Autodesk Inventor part; units mm, degrees
ref_plane "YZ Plane" through (0, 0, 0) normal (1, 0, 0) x (0, 1, 0)
ref_plane "XZ Plane" through (0, 0, 0) normal (0, 1, 0) x (-1, 0, 0)
ref_plane "XY Plane" through (0, 0, 0) normal (0, 0, 1) x (1, 0, 0)
sketch "Sketch1" plane through (0, 0, 0) normal (0, 0, 1) x (1, 0, 0)
  line L0 (-7.182, 9.0471) -> (3.8416, 9.0471)
  line L1 (3.8416, 9.0471) -> (3.8416, -44.5723)
  line L2 (3.8416, -44.5723) -> (-7.182, -44.5723)
  line L3 (-7.182, -44.5723) -> (-7.182, 9.0471)
  point P0 (0, 0)
  dimension "d0" = 11.0236
  dimension "d1" = 53.6194
extrude "Extrusion1" add sketch "Sketch1" along normal blind 1.7018
sketch "Sketch2" plane through (0, 0, 1.7018) normal (0, 0, 1) x (1, 0, 0)
  line L0 (3.8416, 9.0471) -> (-7.182, 9.0471)
  line L1 (3.8416, -44.5723) -> (3.8416, 9.0471)
  line L2 (-7.182, 9.0471) -> (3.8416, 9.0471)
  line L3 (3.8416, 9.0471) -> (3.8416, -15.0829)
  line L4 (3.8416, -15.0829) -> (-7.182, -15.0829)
  line L5 (-7.182, -15.0829) -> (-7.182, 9.0471)
  point P0 (0, 0)
  dimension "d4" = 24.13
extrude "Extrusion2" add sketch "Sketch2" along normal blind 13.843
sketch "Sketch3" plane through (-7.182, 9.0471, 0) normal (0, 1, 0) x (1, 0, 0)
  circle A0 centre (5.5118, -11.3348) radius 1.5
  line L0 (11.0236, -15.5448) -> (0, -15.5448)
  point P0 (7.182, 0)
  dimension "d7" = 3
  dimension "d8" = 4.21
extrude "Extrusion3" cut sketch "Sketch3" against normal blind 25.4
chamfer "Chamfer1" distance 12.7 angle 45 1 edges at (-1.6702, 9.0471, 15.5448)
sketch "Sketch4" plane through (-7.182, 9.0471, 0) normal (0, 1, 0) x (1, 0, 0)
  line L0 (11.0236, -2.8448) -> (0, -2.8448)
  line L1 (0, -15.5448) -> (11.0236, -15.5448)
  line L2 (1.7272, -2.8448) -> (9.2964, -2.8448)
  line L3 (9.2964, -2.8448) -> (9.2964, -15.5448)
  line L4 (9.2964, -15.5448) -> (1.7272, -15.5448)
  line L5 (1.7272, -15.5448) -> (1.7272, -2.8448)
  point P0 (7.182, 0)
  dimension "d14" = 1.7272
  dimension "d15" = 1.7272
extrude "Extrusion4" cut sketch "Sketch4" against normal blind 22.4028
sketch "Sketch5" plane through (0, 0, 1.7018) normal (0, 0, 1) x (1, 0, 0)
  line L0 (-7.182, -44.5723) -> (3.8416, -44.5723)
  line L1 (3.8416, 9.0471) -> (3.8416, -44.5723)
  line L2 (-7.182, -44.5723) -> (3.8416, -44.5723)
  line L3 (3.8416, -44.5723) -> (3.8416, -20.4423)
  line L4 (3.8416, -20.4423) -> (-7.182, -20.4423)
  line L5 (-7.182, -20.4423) -> (-7.182, -44.5723)
  point P0 (0, 0)
  dimension "d18" = 24.13
extrude "Extrusion5" add sketch "Sketch5" along normal blind 13.843
sketch "Sketch6" plane through (-7.182, -44.5723, 0) normal (0, -1, 0) x (1, 0, 0)
  circle A0 centre (5.5118, 11.3348) radius 1.5
  circle A1 centre (5.5118, 11.3348) radius 1.5
  point P0 (7.182, 0)
extrude "Extrusion6" cut sketch "Sketch6" against normal blind 39.243
chamfer "Chamfer2" distance 12.7 angle 45 1 edges at (-1.6702, -44.5723, 15.5448)
sketch "Sketch7" plane through (-7.182, -44.5723, 0) normal (0, -1, 0) x (1, 0, 0)
  line L0 (1.7272, 2.8448) -> (9.2964, 2.8448)
  line L1 (9.2964, 2.8448) -> (9.2964, 15.5448)
  line L2 (9.2964, 15.5448) -> (1.7272, 15.5448)
  line L3 (9.2964, 2.8448) -> (1.7272, 2.8448)
  line L4 (1.7272, 2.8448) -> (1.7272, 15.5448)
  line L5 (1.7272, 15.5448) -> (9.2964, 15.5448)
  line L6 (9.2964, 15.5448) -> (9.2964, 2.8448)
  point P0 (7.182, 0)
extrude "Extrusion7" cut sketch "Sketch7" against normal blind 22.4028
sketch "Sketch8" plane through (-5.4548, -44.5723, 2.8448) normal (0, 0, 1) x (1, 0, 0)
  circle A0 centre (3.7846, 11.2014) radius 1.5
  circle A1 centre (3.7846, 42.418) radius 1.5034
  line L0 (0, 0) -> (7.5692, 0)
  line L1 (7.5692, 53.6194) -> (0, 53.6194)
  point P0 (5.4548, 44.5723)
  dimension "d28" = 3
  dimension "d29" = 3.0067
  dimension "d30" = 11.2014
  dimension "d31" = 11.2014
extrude "Extrusion8" cut sketch "Sketch8" against normal blind 22.4028
fillet "Fillet1" radius 5.08 4 edges at (-7.182, 9.0471, 1.4224) (3.8416, 9.0471, 1.4224) (-7.182, -44.5723, 1.4224) (3.8416, -44.5723, 1.4224)
equation "\"d31\" = d30"
properties part number "Control board Holder"
Work out the finished part from the listing and answer in its coordinate system (mm). A direction names the side the tool comes from. Give positions to 0.01 mm unless a question says otherwise; leave off trailing zeros. Order: outer loops, then holes, each group sorted by start corner. A loop starts at its lowest first (then second) coordinate and runs counter-clockwise, first axis right, second up. Notation, with made-up numbers: M -15.5,29 L 0.5,29 A25 ccw 0.5,65 Z; hole C 82.5,19.5 d8. An arc over 180 degrees is marked long. Return JSON: item names as keys, results as strings.
Q1. Find section D-D, the plane x = 0.5. Write down the section's boundary in (y, z), and give its area (3 significant figures).
Answer below:
{"outline": "M -44.27,0 L 8.74,0 L 8.74,2.84 L -13.36,2.84 L -13.36,15.54 L -15.08,15.54 L -15.08,1.7 L -20.44,1.7 L -20.44,15.54 L -22.17,15.54 L -22.17,2.84 L -44.27,2.84 Z", "area": "189 mm^2"}
Q2. Each of these flat-tipped pins is pushed along its axis until it touches: pin 1 (6 mm diameter, centred on x = -3.5, y = -1, fed in from +Z); pin 2 (5 mm diameter, centred on x = -1.67, z = 11.33, fed in from +Y); pin 3 (5 mm diameter, centred on x = 0.5, z = 5, fed in from -Y). Where does it stop, or does it pass through?
Answer below:
{"pin 1": "stops at z = 15.17", "pin 2": "stops at y = -13.36", "pin 3": "stops at y = -44.55"}
Q3. Find section A-A, the plane z = 2.25. Write down the section's boundary in (x, y).
Answer below:
{"outline": "M -7.18,-39.49 A5.08 ccw -2.1,-44.57 L -1.24,-44.57 A5.08 ccw 3.84,-39.49 L 3.84,-20.44 L -7.18,-20.44 Z; M -7.18,-15.08 L 3.84,-15.08 L 3.84,3.97 A5.08 ccw -1.24,9.05 L -2.1,9.05 A5.08 ccw -7.18,3.97 Z; hole C -1.67,-33.37 d3; hole C -1.67,-2.15 d3.01"}
Q4. The mould has two halves that part along X. Classify faces 1 (the face through (-5.455, -5, 8)), 2 (the face through (-1.995, -34.835, 1.442)), 3 (the face through (2.966, -37.51, 9.907)), 4 (the face through (2.955, 6.835, 2.257)): pulls with the +X half, pulls with the -X half, needs draft (parallel to the pull), parting line crosses it, or undercut.
Answer below:
{"face 1": "undercut", "face 2": "undercut", "face 3": "needs draft", "face 4": "pulls with the +X half"}
Q5. Which of the six approach directions +Z, -Z, +X, -X, +Y, -Y give full straight-line access (tool end or side, diameter ignored) to faces 5 (the face through (-5.455, -31, 8)), 6 (the face through (-2, -20.442, 9)), 7 (the face through (2.114, -5, 8))?
Answer below:
{"face 5": "+Z, -Y", "face 6": "+Z, +X, -X", "face 7": "+Z, +Y"}
Q6. Find section B-B, the plane y = -12. Write down the section's boundary in (x, z).
Answer below:
{"outline": "M -7.18,0 L 3.84,0 L 3.84,15.54 L 2.11,15.54 L 2.11,2.84 L -5.45,2.84 L -5.45,15.54 L -7.18,15.54 Z"}
Q7. Find the intervals of material crossed by line 1 along Y through (x, z) = (1, 4); line 2 along X through (y, z) = (-30, 7.75); line 3 along Z through (x, y) = (-5.25, -33.5), in increasing order. Write a range as [from, to].
Answer below:
{"line 1": "y = [-22.17, -20.44], [-15.08, -13.36]", "line 2": "x = [-7.18, -5.45], [2.11, 3.84]", "line 3": "z = [0, 2.84]"}
Q8. Find section C-C, the plane z = 13.5. Write down the section's boundary in (x, y).
Answer below:
{"outline": "M -7.18,-33.92 L -5.45,-33.92 L -5.45,-22.17 L 2.11,-22.17 L 2.11,-33.92 L 3.84,-33.92 L 3.84,-20.44 L -7.18,-20.44 Z; M -7.18,-15.08 L 3.84,-15.08 L 3.84,-1.61 L 2.11,-1.61 L 2.11,-13.36 L -5.45,-13.36 L -5.45,-1.61 L -7.18,-1.61 Z"}
